from build123d import *

# Parameters (mm, degrees)
F0_R     = 3
F1_DEPTH = 10.5
F2_R     = 1.1
F3_DEPTH = 1.5
F4_W     = 13.6
F4_H     = 9
F5_DEPTH = 25
F6_R     = 1.2


with BuildPart() as f1:
    # F0 (on Top) → F1 (new body)
    with BuildSketch(Plane.XY):
        Polygon((7, 6.313708), (-7, 6.313708), (-8.3, 6.313708), (-8.3, -6.313708), (-7, -6.313708), (7, -6.313708), (8.3, -6.313708), (8.3, 6.313708), align=None)
        Circle(F0_R, mode=Mode.SUBTRACT)
        Circle(F0_R)
    extrude(amount=-F1_DEPTH)

    # F2 (on face) + F0 (on Top) → F3 (join)
    with BuildSketch(Plane.XY):
        with BuildLine():
            ThreePointArc((-20.860771, -16.61813), (-23.399578, -16.804495), (-24.211556, -19.217162))
            Line((-24.211556, -19.217162), (-23.843491, -20.5908))
            Line((-23.843491, -20.5908), (-24.849064, -21.596373))
            ThreePointArc((-24.849064, -21.596373), (-24.849064, -24.849064), (-21.596373, -24.849064))
            Line((-21.596373, -24.849064), (-20.5908, -23.843491))
            Line((-20.5908, -23.843491), (-19.217162, -24.211556))
            ThreePointArc((-19.217162, -24.211556), (-16.804495, -23.399578), (-16.61813, -20.860771))
            Line((-16.61813, -20.860771), (-7.071068, -11.313708))
            ThreePointArc((-7.071068, -11.313708), (0, -8.384776), (7.071068, -11.313708))
            Line((7.071068, -11.313708), (16.61813, -20.860771))
            ThreePointArc((16.61813, -20.860771), (16.804495, -23.399578), (19.217162, -24.211556))
            Line((19.217162, -24.211556), (20.5908, -23.843491))
            Line((20.5908, -23.843491), (21.596373, -24.849064))
            ThreePointArc((21.596373, -24.849064), (24.849064, -24.849064), (24.849064, -21.596373))
            Line((24.849064, -21.596373), (23.843491, -20.5908))
            Line((23.843491, -20.5908), (24.211556, -19.217162))
            ThreePointArc((24.211556, -19.217162), (23.399578, -16.804495), (20.860771, -16.61813))
            Line((20.860771, -16.61813), (11.313708, -7.071068))
            ThreePointArc((11.313708, -7.071068), (8.384776, 0), (11.313708, 7.071068))
            Line((11.313708, 7.071068), (20.860771, 16.61813))
            ThreePointArc((20.860771, 16.61813), (23.399578, 16.804495), (24.211556, 19.217162))
            Line((24.211556, 19.217162), (23.843491, 20.5908))
            Line((23.843491, 20.5908), (24.849064, 21.596373))
            ThreePointArc((24.849064, 21.596373), (24.849064, 24.849064), (21.596373, 24.849064))
            Line((21.596373, 24.849064), (20.5908, 23.843491))
            Line((20.5908, 23.843491), (19.217162, 24.211556))
            ThreePointArc((19.217162, 24.211556), (16.804495, 23.399578), (16.61813, 20.860771))
            Line((16.61813, 20.860771), (7.071068, 11.313708))
            ThreePointArc((7.071068, 11.313708), (0, 8.384776), (-7.071068, 11.313708))
            Line((-7.071068, 11.313708), (-16.61813, 20.860771))
            ThreePointArc((-16.61813, 20.860771), (-16.804495, 23.399578), (-19.217162, 24.211556))
            Line((-19.217162, 24.211556), (-20.5908, 23.843491))
            Line((-20.5908, 23.843491), (-21.596373, 24.849064))
            ThreePointArc((-21.596373, 24.849064), (-24.849064, 24.849064), (-24.849064, 21.596373))
            Line((-24.849064, 21.596373), (-23.843491, 20.5908))
            Line((-23.843491, 20.5908), (-24.211556, 19.217162))
            ThreePointArc((-24.211556, 19.217162), (-23.399578, 16.804495), (-20.860771, 16.61813))
            Line((-20.860771, 16.61813), (-11.313708, 7.071068))
            ThreePointArc((-11.313708, 7.071068), (-8.384776, 0), (-11.313708, -7.071068))
            Line((-11.313708, -7.071068), (-20.860771, -16.61813))
        make_face()
        with BuildLine():
            ThreePointArc((-18.414823, -21.217186), (-17.849138, -22.196982), (-18.828934, -22.762668))
            Line((-18.828934, -22.762668), (-20.939524, -22.197137))
            ThreePointArc((-20.939524, -22.197137), (-21.031939, -22.197137), (-21.111973, -22.243344))
            Line((-21.111973, -22.243344), (-22.657033, -23.788404))
            ThreePointArc((-22.657033, -23.788404), (-23.788404, -23.788404), (-23.788404, -22.657033))
            Line((-23.788404, -22.657033), (-22.243344, -21.111973))
            ThreePointArc((-22.243344, -21.111973), (-22.197137, -21.031939), (-22.197137, -20.939524))
            Line((-22.197137, -20.939524), (-22.762668, -18.828934))
            ThreePointArc((-22.762668, -18.828934), (-22.196982, -17.849138), (-21.217186, -18.414823))
            Line((-21.217186, -18.414823), (-20.651655, -20.525414))
            ThreePointArc((-20.651655, -20.525414), (-20.605448, -20.605448), (-20.525414, -20.651655))
            Line((-20.525414, -20.651655), (-18.414823, -21.217186))
        make_face(mode=Mode.SUBTRACT)
        with Locations((-8, -8)):
            Circle(F2_R, mode=Mode.SUBTRACT)
        with BuildLine():
            Line((22.657033, -23.788404), (21.111973, -22.243344))
            ThreePointArc((21.111973, -22.243344), (21.031939, -22.197137), (20.939524, -22.197137))
            Line((20.939524, -22.197137), (18.828934, -22.762668))
            ThreePointArc((18.828934, -22.762668), (17.849138, -22.196982), (18.414823, -21.217186))
            Line((18.414823, -21.217186), (20.525414, -20.651655))
            ThreePointArc((20.525414, -20.651655), (20.605448, -20.605448), (20.651655, -20.525414))
            Line((20.651655, -20.525414), (21.217186, -18.414823))
            ThreePointArc((21.217186, -18.414823), (22.196982, -17.849138), (22.762668, -18.828934))
            Line((22.762668, -18.828934), (22.197137, -20.939524))
            ThreePointArc((22.197137, -20.939524), (22.197137, -21.031939), (22.243344, -21.111973))
            Line((22.243344, -21.111973), (23.788404, -22.657033))
            ThreePointArc((23.788404, -22.657033), (23.788404, -23.788404), (22.657033, -23.788404))
        make_face(mode=Mode.SUBTRACT)
        with Locations((8, -8)):
            Circle(F2_R, mode=Mode.SUBTRACT)
        with Locations((-8, 8)):
            Circle(F2_R, mode=Mode.SUBTRACT)
        with BuildLine():
            Line((-22.657033, 23.788404), (-21.111973, 22.243344))
            ThreePointArc((-21.111973, 22.243344), (-21.031939, 22.197137), (-20.939524, 22.197137))
            Line((-20.939524, 22.197137), (-18.828934, 22.762668))
            ThreePointArc((-18.828934, 22.762668), (-17.849138, 22.196982), (-18.414823, 21.217186))
            Line((-18.414823, 21.217186), (-20.525414, 20.651655))
            ThreePointArc((-20.525414, 20.651655), (-20.605448, 20.605448), (-20.651655, 20.525414))
            Line((-20.651655, 20.525414), (-21.217186, 18.414823))
            ThreePointArc((-21.217186, 18.414823), (-22.196982, 17.849138), (-22.762668, 18.828934))
            Line((-22.762668, 18.828934), (-22.197137, 20.939524))
            ThreePointArc((-22.197137, 20.939524), (-22.197137, 21.031939), (-22.243344, 21.111973))
            Line((-22.243344, 21.111973), (-23.788404, 22.657033))
            ThreePointArc((-23.788404, 22.657033), (-23.788404, 23.788404), (-22.657033, 23.788404))
        make_face(mode=Mode.SUBTRACT)
        Polygon((-8.3, -6.313708), (-8.3, 6.313708), (-7, 6.313708), (7, 6.313708), (8.3, 6.313708), (8.3, -6.313708), (7, -6.313708), (-7, -6.313708), align=None, mode=Mode.SUBTRACT)
        with Locations((8, 8)):
            Circle(F2_R, mode=Mode.SUBTRACT)
        with BuildLine():
            Line((23.788404, 22.657033), (22.243344, 21.111973))
            ThreePointArc((22.243344, 21.111973), (22.197137, 21.031939), (22.197137, 20.939524))
            Line((22.197137, 20.939524), (22.762668, 18.828934))
            ThreePointArc((22.762668, 18.828934), (22.196982, 17.849138), (21.217186, 18.414823))
            Line((21.217186, 18.414823), (20.651655, 20.525414))
            ThreePointArc((20.651655, 20.525414), (20.605448, 20.605448), (20.525414, 20.651655))
            Line((20.525414, 20.651655), (18.414823, 21.217186))
            ThreePointArc((18.414823, 21.217186), (17.849138, 22.196982), (18.828934, 22.762668))
            Line((18.828934, 22.762668), (20.939524, 22.197137))
            ThreePointArc((20.939524, 22.197137), (21.031939, 22.197137), (21.111973, 22.243344))
            Line((21.111973, 22.243344), (22.657033, 23.788404))
            ThreePointArc((22.657033, 23.788404), (23.788404, 23.788404), (23.788404, 22.657033))
        make_face(mode=Mode.SUBTRACT)
    with BuildSketch(Plane.XY):
        Polygon((7, 6.313708), (-7, 6.313708), (-8.3, 6.313708), (-8.3, -6.313708), (-7, -6.313708), (7, -6.313708), (8.3, -6.313708), (8.3, 6.313708), align=None)
        Circle(F0_R, mode=Mode.SUBTRACT)
    extrude(amount=F3_DEPTH)

    # F4 (on face) → F5 (cut)
    with BuildSketch(Plane.XZ.offset(6.313708)):
        with Locations((0, -4.5)):
            Rectangle(F4_W, F4_H)
    extrude(amount=-F5_DEPTH, mode=Mode.SUBTRACT)

    # F6
    f6_edges = [f1.edges().sort_by_distance(p)[0] for p in [
        (8.3, 0, -10.5),
        (-8.3, 0, -10.5),
        (-6.8, 0, -9),
        (6.8, 0, -9),
    ]]
    fillet(f6_edges, radius=F6_R)


solid = f1.part
Model file for the job. Use its own axes, mm. A direction names the side the tool comes from. Round coordinates to 2 decimals unless told otherwise and drop trailing zeros. Order: outer loops, then holes, each group sorted by start corner. A loop starts at its lowest first (then second) coordinate and runs counter-clockwise, first axis right, second up.
(1) Pin check, flat tips, straight feed: pin 1 (5 mm diameter, centred on x = 11, z = -4, fed in from +Y); pin 2 (10 mm diameter, centred on x = 19, y = 17.5, fed in from -Z); pin 3 (5 mm diameter, centred on y = 20, z = -0.5, fed in from -X); pin 4 (6 mm diameter, centred on y = 2.5, z = -3.5, fed in from -X). Stop position of each tip, or through.
(2) Band-saw the part on A-A (z = -2). List the corners of the cut face in (x, y), then the cut area to 3 significant figures.
(3) Drill centre lines: line 1 (Y direction, x = 0, z = 0.35); line 2 (Y direction, x = 8, z = 0.4); line 3 (Z direction, x = 5, y = -5). Where is each one in solid material? Low to high.
(4) 3-axis set-ups, long thin cutter, end or side, ignore diameter. For faces 4 (the face through (-3, 0, 1)), 5 (the face through (1, 6.314, -10)), 6 (the face through (20, -24, 1)), 7 (the face through (19.869, 22.484, 0.74)): which of +Z, -Z, +X, -X, +Y, -Y reach the whole face in a straight line?
(5) Band-saw the part on B-B (x = 0). List the corners of the cut face in (y, z).
(6) Band-saw the part on C-C (y = 15). List the corners of the cut face in (x, z).
(7) Band-saw the part on D-D (y = -1). List the corners of the cut face in (x, z).
(8) Pull direction X, two halves, no side cores. Call faces 1 (the face through (8.3, 0, -5)), 2 (the face through (-7.939, -0.088, -10.158)), 3 (the face through (-24.884, -24.813, 0.74)): released by +X, released by -X, zero draft, split by the parting line, or undercut.
Verdict:
1. pin 1: passes through
1. pin 2: stops at z = 0
1. pin 3: stops at x = -25.39
1. pin 4: stops at x = -8.3
2. outline: (-8.3, -6.31) - (-6.8, -6.31) - (-6.8, 6.31) - (-8.3, 6.31) - close; (6.8, -6.31) - (8.3, -6.31) - (8.3, 6.31) - (6.8, 6.31) - close
2. area: 37.9 mm2
3. line 1: y = -8.38 to -3, 3 to 8.38
3. line 2: y = -12.24 to -9.1, -6.9 to 6.9, 9.1 to 12.24
3. line 3: z = -10.5 to -9, 0 to 1.5
4. face 4: +Z
4. face 5: -Z, +X, -X, +Y
4. face 6: +Z, -Z, -Y
4. face 7: +Z, -Z
5. outline: (-8.38, 0) - (-3, 0) - (-3, 1.5) - (-8.38, 1.5) - close; (-6.31, -10.5) - (6.31, -10.5) - (6.31, -9) - (-6.31, -9) - close; (3, 0) - (8.38, 0) - (8.38, 1.5) - (3, 1.5) - close
6. outline: (-19.24, 0) - (-10.76, 0) - (-10.76, 1.5) - (-19.24, 1.5) - close; (10.76, 0) - (19.24, 0) - (19.24, 1.5) - (10.76, 1.5) - close
7. outline: (-8.43, 0) - (-8.3, 0) - (-8.3, -9.3) arc R1.2 ccw to (-7.1, -10.5) - (7.1, -10.5) arc R1.2 ccw to (8.3, -9.3) - (8.3, 0) - (8.43, 0) - (8.43, 1.5) - (2.83, 1.5) - (2.83, 0) - (6.8, 0) - (6.8, -7.8) arc R1.2 cw to (5.6, -9) - (-5.6, -9) arc R1.2 cw to (-6.8, -7.8) - (-6.8, 0) - (-2.83, 0) - (-2.83, 1.5) - (-8.43, 1.5) - close
8. face 1: released by +X
8. face 2: released by -X
8. face 3: undercut
